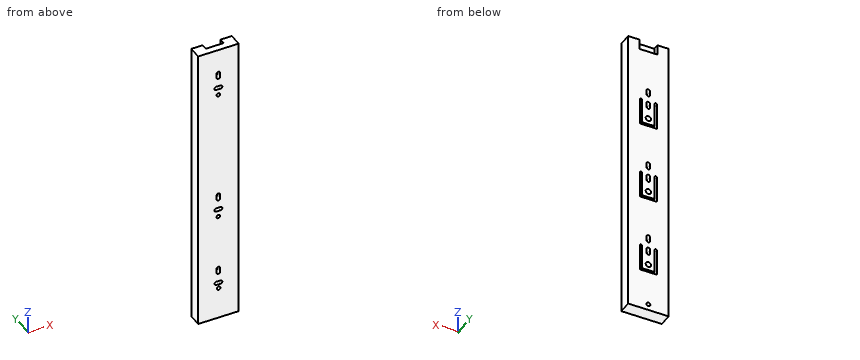
Autodesk Inventor part; units mm, degrees
ref_plane "YZ Plane" through (0, 0, 0) normal (1, 0, 0) x (0, 1, 0)
ref_plane "XZ Plane" through (0, 0, 0) normal (0, 1, 0) x (-1, 0, 0)
ref_plane "XY Plane" through (0, 0, 0) normal (0, 0, 1) x (1, 0, 0)
sketch "Sketch1" plane through (0, 0, 0) normal (0, 1, 0) x (-1, 0, 0)
  line L0 (-23.9141, 174.625) -> (23.9141, 174.625)
  line L1 (23.9141, 174.625) -> (23.9141, -174.625)
  line L2 (23.9141, -174.625) -> (-23.9141, -174.625)
  line L3 (-23.9141, -174.625) -> (-23.9141, 174.625)
  line L4 (-23.9141, 174.625) -> (23.9141, -174.625) construction
  line L5 (23.9141, 174.625) -> (-23.9141, -174.625) construction
  point P0 (0, 0)
  dimension "d0" = 47.8282
  dimension "d1" = 349.25
extrude "Extrusion1" add sketch "Sketch1" along normal blind 15.0622
sketch "Sketch2" plane through (0, 15.0622, 0) normal (0, 1, 0) x (1, 0, 0)
  line L0 (-10.6299, -174.625) -> (10.6426, -174.625)
  line L1 (10.6426, -174.625) -> (10.6426, -162.4584)
  line L2 (10.6426, -162.4584) -> (-10.6299, -162.4584)
  line L3 (-10.6299, -162.4584) -> (-10.6299, -174.625)
  line L4 (-23.9141, -174.625) -> (23.9141, -174.625)
  line L5 (-23.9141, 174.625) -> (-23.9141, -174.625)
  point P0 (0, 0)
  point P1 (0, -132.6268)
  dimension "d4" = 21.2725
  dimension "d5" = 12.1666
  dimension "d6" = 13.2842
  dimension "d7" = 23.9141
extrude "Extrusion2" cut sketch "Sketch2" against normal blind 6.858
sketch "Sketch3" plane through (0, 15.0622, 0) normal (0, 1, 0) x (1, 0, 0)
  circle A0 centre (0, -111.252) radius 2.1336
  line L0 (-10.6299, -162.4584) -> (10.6426, -162.4584)
  circle A1 centre (0.0065, -106.299) radius 2.1336
  line L1 (-2.1271, -106.2962) -> (-2.1336, -111.2492)
  line L2 (2.1401, -106.3018) -> (2.1336, -111.2548)
  line L3 (0.0064, -93.8649) -> (0.0064, -74.1654) construction
  circle A2 centre (0, -94.9706) radius 2.1336
  circle A3 centre (0.0065, -90.0176) radius 2.1336
  line L4 (-2.1271, -90.0148) -> (-2.1336, -94.9678)
  line L5 (2.1401, -90.0204) -> (2.1336, -94.9734)
  circle A4 centre (0, -16.002) radius 2.1336
  circle A5 centre (0.0065, -11.049) radius 2.1336
  line L6 (-2.1271, -11.0462) -> (-2.1336, -15.9992)
  line L7 (2.1401, -11.0518) -> (2.1336, -16.0048)
  circle A6 centre (0, 0.2794) radius 2.1336
  circle A7 centre (0.0065, 5.2324) radius 2.1336
  line L8 (-2.1271, 5.2352) -> (-2.1336, 0.2822)
  line L9 (2.1401, 5.2296) -> (2.1336, 0.2766)
  circle A8 centre (0, 79.248) radius 2.1336
  circle A9 centre (0.0065, 84.201) radius 2.1336
  line L10 (-2.1271, 84.2038) -> (-2.1336, 79.2508)
  line L11 (2.1401, 84.1982) -> (2.1336, 79.2452)
  circle A10 centre (0, 95.5294) radius 2.1336
  circle A11 centre (0.0065, 100.4824) radius 2.1336
  line L12 (-2.1271, 100.4852) -> (-2.1336, 95.5322)
  line L13 (2.1401, 100.4796) -> (2.1336, 95.5266)
  point P0 (0, 0)
  point P1 (0.0064, 1.3851)
  point P2 (0.0064, 96.6351)
  dimension "d10" = 4.2672
  dimension "d11" = 51.2064
  dimension "d12" = 4.2672
  dimension "d13" = 9.2202
  dimension "d18" = 16.2814
  dimension "d34" = 95.25
sketch "Sketch4" plane through (0, 15.0622, 0) normal (0, 1, 0) x (1, 0, 0)
  line L0 (-9.9568, -97.1042) -> (-9.9568, -65.3542)
  line L1 (-9.9568, -65.3542) -> (9.9568, -65.3542)
  line L2 (9.9568, -65.3542) -> (9.9568, -97.1042)
  arc A0 (-2.1336, -111.2492) -> (2.1336, -111.2548) centre (0, -111.252) ccw construction
  line L3 (-7.4168, -97.1042) -> (-7.4168, -67.8942)
  line L4 (-7.4168, -67.8942) -> (7.4168, -67.8942)
  line L5 (7.4168, -67.8942) -> (7.4168, -97.2756)
  line L6 (-16.8514, -97.1042) -> (16.8246, -97.1042) construction
  arc A1 (-2.1336, -94.9678) -> (2.1336, -94.9734) centre (0, -94.9706) ccw construction
  arc A2 (-9.9568, -97.1042) -> (-7.4168, -97.1042) centre (-8.6868, -97.1042) ccw
  arc A3 (7.4168, -97.2756) -> (9.9568, -97.1042) centre (8.6926, -97.2756) ccw
  circle A4 centre (0, -75.2158) radius 3.175
  line L7 (0, 24.1867) -> (0, 36.4789) construction
  arc A5 (-9.9568, -1.8542) -> (-7.4168, -1.8542) centre (-8.6868, -1.8542) ccw
  arc A6 (7.4168, -2.0256) -> (9.9568, -1.8542) centre (8.6926, -2.0256) ccw
  circle A7 centre (0, 20.0342) radius 3.175
  line L8 (-7.4168, -1.8542) -> (-7.4168, 27.3558)
  line L9 (7.4168, 27.3558) -> (7.4168, -2.0256)
  line L10 (-7.4168, 27.3558) -> (7.4168, 27.3558)
  line L11 (-9.9568, 29.8958) -> (9.9568, 29.8958)
  line L12 (9.9568, 29.8958) -> (9.9568, -1.8542)
  line L13 (-9.9568, -1.8542) -> (-9.9568, 29.8958)
  arc A8 (-9.9568, 93.3958) -> (-7.4168, 93.3958) centre (-8.6868, 93.3958) ccw
  arc A9 (7.4168, 93.2244) -> (9.9568, 93.3958) centre (8.6926, 93.2244) ccw
  circle A10 centre (0, 115.2842) radius 3.175
  line L14 (-7.4168, 93.3958) -> (-7.4168, 122.6058)
  line L15 (7.4168, 122.6058) -> (7.4168, 93.2244)
  line L16 (-7.4168, 122.6058) -> (7.4168, 122.6058)
  line L17 (-9.9568, 125.1458) -> (9.9568, 125.1458)
  line L18 (9.9568, 125.1458) -> (9.9568, 93.3958)
  line L19 (-9.9568, 93.3958) -> (-9.9568, 125.1458)
  point P0 (0, 0)
  point P1 (16.8246, -1.8542)
  point P2 (16.8246, 93.3958)
  dimension "d25" = 31.75
  dimension "d26" = 19.9136
  dimension "d28" = 9.9568
  dimension "d29" = 2.54
  dimension "d30" = 0
  dimension "d31" = 6.35
  dimension "d41" = 95.25
extrude "Extrusion5" cut sketch "Sketch4" against normal blind 6.858
extrude "Extrusion6" cut sketch "Sketch3" against normal blind 6.858
sketch "Sketch5" plane through (0, 15.0622, 0) normal (0, 1, 0) x (1, 0, 0)
  circle A0 centre (0, 167.3174) radius 2.3546
  line L0 (23.9141, 174.625) -> (-23.9141, 174.625)
  point P0 (0, 0)
  dimension "d50" = 4.7092
  dimension "d51" = 4.953
extrude "Extrusion7" cut sketch "Sketch5" against normal blind 6.858
sketch "Sketch6" plane through (0, 0, 0) normal (0, -1, 0) x (1, 0, 0)
  circle A0 centre (0, 144.0685) radius 2.159
  circle A1 centre (0, 139.1358) radius 2.159
  line L0 (2.159, 144.0685) -> (2.159, 139.1358)
  line L1 (-2.159, 144.0685) -> (-2.159, 139.1358)
  line L2 (2.4765, 127.6296) -> (-2.4765, 127.6296)
  circle A2 centre (2.4765, 125.4706) radius 2.159
  circle A3 centre (-2.4765, 125.4706) radius 2.159
  line L3 (-0.0635, 119.2045) -> (-0.0635, 135.9892) construction
  line L4 (23.9141, -174.625) -> (23.9141, 174.625)
  line L5 (2.4765, 123.3116) -> (-2.4765, 123.3116)
  line L6 (-23.9141, 174.625) -> (-23.9141, -174.625)
  circle A4 centre (0, 116.0726) radius 2.159
  line L7 (0, 93.2461) -> (0, 84.503) construction
  line L8 (2.4765, -35.4384) -> (-2.4765, -35.4384)
  circle A5 centre (2.4765, -33.2794) radius 2.159
  circle A6 centre (-2.4765, -33.2794) radius 2.159
  circle A7 centre (0, -19.6142) radius 2.159
  circle A8 centre (0, -42.6774) radius 2.159
  line L9 (2.159, -14.6815) -> (2.159, -19.6142)
  line L10 (-2.159, -14.6815) -> (-2.159, -19.6142)
  line L11 (-0.0635, -39.5455) -> (-0.0635, -22.7608) construction
  line L12 (2.4765, -31.1204) -> (-2.4765, -31.1204)
  circle A9 centre (0, -14.6815) radius 2.159
  line L13 (0, -44.8364) -> (0, -108.3364) construction
  point P0 (0, 0)
  dimension "d54" = 4.318
  dimension "d55" = 4.318
  dimension "d56" = 9.2507
  dimension "d61" = 9.3472
  dimension "d62" = 4.318
  dimension "d63" = 4.318
  dimension "d64" = 9.271
  dimension "d65" = 19.2786
  dimension "d66" = 23.9141
  dimension "d67" = 4.318
  dimension "d68" = 5.08
  dimension "d71" = 158.75
  dimension "d76" = 63.5
sketch "Sketch7" plane through (0, 0, 0) normal (0, -1, 0) x (1, 0, 0)
  circle A0 centre (0, -110.4954) radius 2.159
  line L0 (23.9141, 174.625) -> (-23.9141, 174.625)
  line L1 (-23.9141, 174.625) -> (-23.9141, -174.625)
  line L2 (-23.9141, -174.625) -> (23.9141, -174.625)
  line L3 (23.9141, -174.625) -> (23.9141, 174.625)
  circle A1 centre (0, -42.6774) radius 2.159
  circle A2 centre (-0.0001, -115.4484) radius 2.159
  line L4 (2.1589, -115.4484) -> (2.159, -110.4955)
  line L5 (-2.159, -115.423) -> (-2.159, -110.4954)
  circle A3 centre (2.4765, -129.1609) radius 2.159
  circle A4 centre (-2.4757, -129.0705) radius 2.159
  line L6 (2.4765, -131.3199) -> (-2.5149, -131.2291)
  line L7 (2.4739, -127.0019) -> (-2.4361, -126.9118)
  circle A5 centre (0.287, -136.3609) radius 2.159
  line L8 (-23.9141, 174.625) -> (-23.9141, -174.625)
  point P0 (0, 0)
  dimension "d79" = 4.318
  dimension "d80" = 63.5
  dimension "d81" = 4.318
  dimension "d82" = 9.271
  dimension "d83" = 4.318
  dimension "d84" = 4.318
  dimension "d85" = 9.271
  dimension "d86" = 21.4376
  dimension "d87" = 9.3472
  dimension "d88" = 4.318
  dimension "d89" = 5.08
extrude "Extrusion10" cut sketch "Sketch6" against normal blind 6.35
extrude "Extrusion11" cut sketch "Sketch7" against normal blind 6.35 contours A0 | L4 A2 L5 A0 | A2 | A3 L6 A4 L7 | A4 | A5
properties part number "drawer rails"
Could you check a few things on this model? Use its own coordinates, in mm. Coordinates: 2 decimals unless noted, no trailing zeros. Answer as CSV lines item,"result". Start each with the question number.
1) Please list where these lines run through material, in increasing order: line 1 (Z direction, x = 5, y = 12) (3 decimals); line 2 (X direction, y = 11.75, z = -106); line 3 (X direction, y = 1, z = -41). Write a range as from..to.
2) For P1, Ø1.9, axis at x = -1, z = -20, coming from the +Y side; P2, Ø4, axis at x = 0, z = 116.07, coming from the -Y side; P3, Ø2, axis at x = 3, y = 12, coming from the +Z side, each with a flat end and sliding along its axis, tell me the tip position at first contact or that it passes through.
3) I want a section at A-A, the plane y = 10.75. Give the number of separate pieces and of enclosed holes in the cut face, and give its area (3 significant figures).
Data:
1,line 1,"z = -174.625..-125.146, -122.606..-29.896, -27.356..65.354, 67.894..162.458"
1,line 2,"x = -23.91..-9.96, -7.42..7.42, 9.96..23.91"
1,line 3,"x = -23.91..-1.36, 1.36..23.91"
2,P1,"stops at y = 8.2"
2,P2,"stops at y = 6.35"
2,P3,"stops at z = 162.46"
3,separate pieces,"1"
3,enclosed holes,"13"
3,area,"15,500 mm^2"
